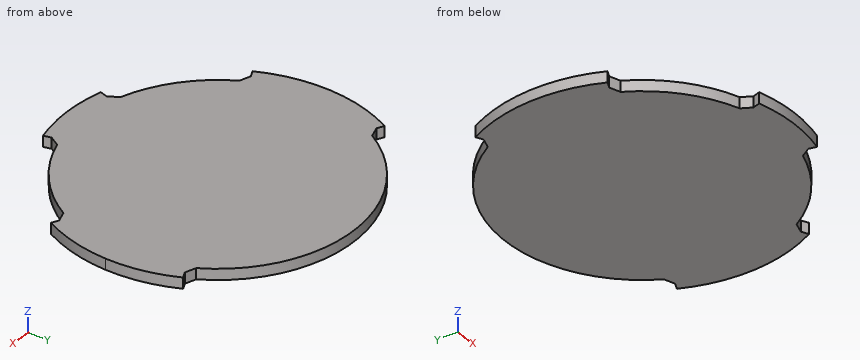
```python
from build123d import *

# Parameters (mm, degrees)
SKETCH1_R           = 44.949380312
BOSS_EXTRUDE1_DEPTH = 3.6


with BuildPart() as part:
    # Sketch1 → Boss-Extrude1 (new body)
    with BuildSketch(Plane.XY):
        with BuildLine():
            Line((-33.14651631, -29.251901051), (-33.785882697, -31.638048893))
            ThreePointArc((-33.785882697, -31.638048893), (-20.906933284, -33.326956191), (-8.027983871, -31.638048893))
            Line((-8.027983871, -31.638048893), (-8.667350258, -29.251901051))
            Line((-8.667350258, -29.251901051), (-6.827368119, -26.064958502))
            ThreePointArc((-6.827368119, -26.064958502), (-20.906933284, -28.326956191), (-34.986498448, -26.064958502))
            Line((-34.986498448, -26.064958502), (-33.14651631, -29.251901051))
        make_face()
        with BuildLine():
            Line((-63.602995354, -4.145517191), (-60.123520772, -5.343596369))
            ThreePointArc((-60.123520772, -5.343596369), (-65.856313596, 16.622424121), (-60.123520772, 38.588444611))
            Line((-60.123520772, 38.588444611), (-63.602995354, 37.390365433))
            Line((-63.602995354, 37.390365433), (-65.823306082, 38.473283331))
            ThreePointArc((-65.823306082, 38.473283331), (-70.856313596, 16.622424121), (-65.823306082, -5.228435089))
            Line((-65.823306082, -5.228435089), (-63.602995354, -4.145517191))
        make_face()
        with BuildLine():
            ThreePointArc((24.042447028, 16.622424121), (22.585641346, 5.271532419), (18.309654204, -5.343596369))
            Line((18.309654204, -5.343596369), (21.789128786, -4.145517191))
            Line((21.789128786, -4.145517191), (24.009439514, -5.228435089))
            ThreePointArc((24.009439514, -5.228435089), (27.767934875, 5.410920956), (29.042447028, 16.622424121))
            ThreePointArc((29.042447028, 16.622424121), (27.767934875, 27.833927286), (24.009439514, 38.473283331))
            Line((24.009439514, 38.473283331), (21.789128786, 37.390365433))
            Line((21.789128786, 37.390365433), (18.309654204, 38.588444611))
            ThreePointArc((18.309654204, 38.588444611), (22.585641346, 27.973315823), (24.042447028, 16.622424121))
        make_face()
        with Locations((-20.906933284, 16.622424121)):
            Circle(SKETCH1_R)
    extrude(amount=BOSS_EXTRUDE1_DEPTH)


solid = part.part
```
The model under review builds one solid part; all positions refer to its coordinate system, in mm. Round coordinates to 2 decimals unless told otherwise and drop trailing zeros. Order: outer loops, then holes, each group sorted by start corner. A loop starts at its lowest first (then second) coordinate and runs counter-clockwise, first axis right, second up.
Item 1: For pin 1 (2 mm diameter, centred on x = -53, z = 3, fed in from +Y); pin 2 (1 mm diameter, centred on y = -22, z = 2, fed in from -X); pin 3 (2 mm diameter, centred on x = -1, z = 3, fed in from -Y), all flat-tipped, find the tip position at first contact; note any pin that passes through.
Working result:
pin 1: stops at y = 49.08
pin 2: stops at x = -44.72
pin 3: stops at y = -24.16
Item 2: Add section C-C, the plane y = 8. State the section outline as (x, z) points, and give its area (3 significant figures).
Working result:
outline: (-70.11, 0) - (28.29, 0) - (28.29, 3.6) - (-70.11, 3.6) - close
area: 354 mm2
Item 3: To check wall thickness, follow probe 1 along X at (y, z) = (18, 2.95); probe 2 along X at (y, z) = (57, 1.75); probe 3 along Y at (x, z) = (-31, 2.6). State the ranges of each line that lie inside material, in increasing order.
Working result:
probe 1: x = -70.84 to 29.02
probe 2: x = -40.66 to -1.16
probe 3: y = -32.3 to 60.42
Item 4: Add section B-B, the plane x = -0.5. State the section outline as (y, z) points.
Working result:
outline: (-23.43, 0) - (56.67, 0) - (56.67, 3.6) - (-23.43, 3.6) - close
Item 5: Add section A-A, the plane z = 0.6. State the section outline as (x, y) points, and give its area (3 significant figures).
Working result:
outline: (-65.82, -5.23) - (-63.6, -4.15) - (-60.12, -5.34) arc R44.95 ccw to (-34.99, -26.06) - (-33.15, -29.25) - (-33.79, -31.64) arc R49.95 ccw to (-8.03, -31.64) - (-8.67, -29.25) - (-6.83, -26.06) arc R44.95 ccw to (18.31, -5.34) - (21.79, -4.15) - (24.01, -5.23) arc R49.95 ccw to (24.01, 38.47) - (21.79, 37.39) - (18.31, 38.59) arc R44.95 ccw to (-60.12, 38.59) - (-63.6, 37.39) - (-65.82, 38.47) arc R49.95 ccw to start
area: 6,920 mm2
